Verification items for the finished model (mm, model axes). Face numbers are marked on the shaded views. A direction names the side the tool comes from. Coordinates: 2 decimals unless noted, no trailing zeros. Order: outer loops, then holes, each group sorted by start corner. A loop starts at its lowest first (then second) coordinate and runs counter-clockwise, first axis right, second up. Notation, with made-up numbers: (51, 63) -> (69, 63) arc R23 cw to (69, 91) -> close; hole circle Ø3 at (83, 46.25). An arc over 180 degrees is marked (long way). Write item = value, one per line. Start each with the question number.
1. Cross-section at A-A on y = 0. Record the cut outline in (x, z), plus the area to 3 significant figures.
2. Cross-section at D-D on x = 19.5. Record the cut outline in (y, z), plus the area to 3 significant figures.
3. Cross-section at B-B on x = 15. Record the cut outline in (y, z), plus the area to 3 significant figures.
4. Go/stop test with flat-tipped pins: P1, Ø5, axis at y = -1, z = -3, coming from the +X side; P2, Ø4, axis at x = -12, y = -2, coming from the -Z side; P3, Ø1.8, axis at x = -3, z = -2, coming from the +Y side. Record where each tip stops, or that it passes through.
5. Thickness scan on line 1 along X through (y, z) = (-1.75, 3.5); line 2 along X through (y, z) = (-3.75, 4.25); line 3 along Y through (x, z) = (8, -1.5). Record the ranges inside material, lowest first. Write a range as from..to.
6. Cross-section at C-C on z = 4. Record the cut outline in (x, y), plus the area to 3 significant figures.
7. Release check for a two-part mould opening along X. For the marked faces 4, 5 and 6 record: +X half, -X half, draft (parallel to the pull), parting line (faces both ways), or undercut.
8. Set-up check for the marked faces 1, 2 and 3: record each of +Z, -Z, +X, -X, +Y, -Y from which the full face is reachable in a straight line by a thin tool's end or side.
from build123d import *

# Parameters (mm, degrees)
SKETCH1_W           = 45
SKETCH1_H           = 12
SKETCH1_R           = 2.15
BOSS_EXTRUDE1_DEPTH = 5
CUT_EXTRUDE1_DEPTH  = 24.817010728
SKETCH3_W           = 18
SKETCH3_H           = 9.5
BOSS_EXTRUDE2_DEPTH = 6
FILLET1_R           = 2


with BuildPart() as part:
    # Sketch1 → Boss-Extrude1 (new body)
    with BuildSketch(Plane.XY):
        Rectangle(SKETCH1_W, SKETCH1_H)
        with Locations((-15, 0)):
            Circle(SKETCH1_R, mode=Mode.SUBTRACT)
        with Locations((15, 0)):
            Circle(SKETCH1_R, mode=Mode.SUBTRACT)
    extrude(amount=BOSS_EXTRUDE1_DEPTH)

    # Sketch2 → Cut-Extrude1 (cut, through all)
    with BuildSketch(Plane.XY.offset(5)):
        with BuildLine():
            Line((-12.9, 2), (-12.9, -2))
            ThreePointArc((-12.9, -2), (-15, -4.1), (-17.1, -2))
            Line((-17.1, -2), (-17.1, 2))
            ThreePointArc((-17.1, 2), (-15, 4.1), (-12.9, 2))
        make_face()
        with BuildLine():
            Line((12.9, -2), (12.9, 2))
            ThreePointArc((12.9, 2), (15, 4.1), (17.1, 2))
            Line((17.1, 2), (17.1, -2))
            ThreePointArc((17.1, -2), (15, -4.1), (12.9, -2))
        make_face()
    extrude(amount=-CUT_EXTRUDE1_DEPTH, mode=Mode.SUBTRACT)

    # Sketch3 → Boss-Extrude2 (add)
    with BuildSketch(Plane.XY):
        with Locations((0, -1.25)):
            Rectangle(SKETCH3_W, SKETCH3_H)
    extrude(amount=-BOSS_EXTRUDE2_DEPTH)

    # Fillet1
    fillet1_edges = [part.edges().sort_by_distance(p)[0] for p in [
        (-22.5, 6, 2.5),
        (-22.5, -6, 2.5),
        (22.5, -6, 2.5),
        (22.5, 6, 2.5),
    ]]
    fillet(fillet1_edges, radius=FILLET1_R)


solid = part.part
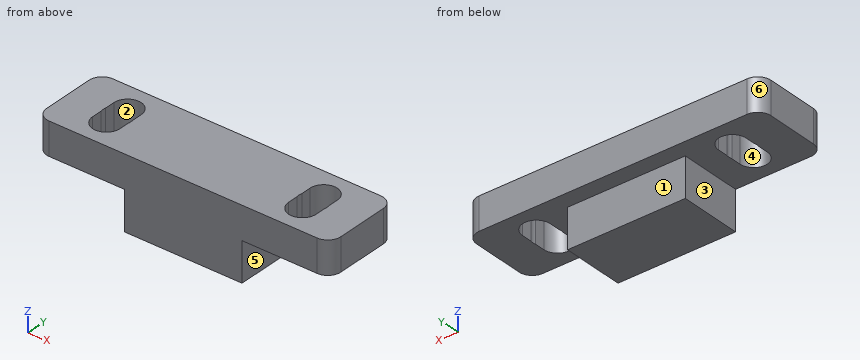
Worked out:
q1.outline = (-22.5, 0) -> (-17.15, 0) -> (-17.15, 5) -> (-22.5, 5) -> close; (-12.85, 0) -> (-9, 0) -> (-9, -6) -> (9, -6) -> (9, 0) -> (12.85, 0) -> (12.85, 5) -> (-12.85, 5) -> close; (17.15, 0) -> (22.5, 0) -> (22.5, 5) -> (17.15, 5) -> close
q1.area = 290 mm²
q2.outline = (-6, 0) -> (6, 0) -> (6, 5) -> (-6, 5) -> close
q2.area = 60.0 mm²
q3.outline = (-6, 0) -> (-4.1, 0) -> (-4.1, 5) -> (-6, 5) -> close; (4.1, 0) -> (6, 0) -> (6, 5) -> (4.1, 5) -> close
q3.area = 19.0 mm²
q4.P1 = 9
q4.P2 = 0
q4.P3 = 3.5
q5.line_1 = -22.5..-17.1, -12.9..12.9, 17.1..22.5
q5.line_2 = -22.5..-16.16, -13.84..13.84, 16.16..22.5
q5.line_3 = -6..3.5
q6.outline = (-22.5, -4) arc R2 ccw to (-20.5, -6) -> (20.5, -6) arc R2 ccw to (22.5, -4) -> (22.5, 4) arc R2 ccw to (20.5, 6) -> (-20.5, 6) arc R2 ccw to (-22.5, 4) -> close; hole (-17.1, -2) arc R2.1 ccw to (-12.9, -2) -> (-12.9, -0.46) arc R2.15 ccw to (-12.9, 0.46) -> (-12.9, 2) arc R2.1 ccw to (-17.1, 2) -> (-17.1, 0.46) arc R2.15 ccw to (-17.1, -0.46) -> close; hole (12.9, -2) arc R2.1 ccw to (17.1, -2) -> (17.1, -0.46) arc R2.15 ccw to (17.1, 0.46) -> (17.1, 2) arc R2.1 ccw to (12.9, 2) -> (12.9, 0.46) arc R2.15 ccw to (12.9, -0.46) -> close
q6.area = 475 mm²
q7.face_4 = undercut
q7.face_5 = +X half
q7.face_6 = -X half
q8.face_1 = -Z, +X, -X, +Y
q8.face_2 = +Z, -Z
q8.face_3 = -Z, -X, +Y, -Y
